Can you work these out from the model? Positions are in its coordinate system, mm. Face numbers are marked on the shaded views. Coordinates: 2 decimals unless noted, no trailing zeros. Loops run counter-clockwise (first coordinate to the right, second up) from the corner with the lowest first, then second, coordinate; pieces in that order, holes last.
```python
from build123d import *

# Parameters (mm, degrees)
SKETCH_1_R      = 13.5
SKETCH_1_R_2    = 10
EXTRUDE_1_DEPTH = 4


with BuildPart() as part:
    # 草图1 → 凸台-拉伸1 (new body)
    with BuildSketch(Plane(origin=(0, 0, 0), x_dir=(1, 0, 0), z_dir=(0, 1, 0))):
        with Locations(Location((0, 0, 0), (0, 0, 270))):
            Circle(SKETCH_1_R)
        with Locations(Location((0, 0, 0), (0, 0, 270))):
            Circle(SKETCH_1_R_2, mode=Mode.SUBTRACT)
    extrude(amount=EXTRUDE_1_DEPTH)

    # 草图3 → 切除-旋转1 (revolve, cut)
    with BuildSketch(Plane.XY, mode=Mode.PRIVATE) as cut_revolve_1_sk:
        Polygon((-12.25, 3.566987298), (-12, 4), (-12.5, 4), align=None)
        Polygon((-10.75, 3.566987298), (-10.5, 4), (-11, 4), align=None)
    cut_revolve_1 = revolve(cut_revolve_1_sk.sketch.rotate(Axis((0, 4, 0), (0, 1, 0)), 270), axis=Axis((0, 4, 0), (0, 1, 0)), mode=Mode.SUBTRACT)

    # 镜向1: 切除-旋转1 across plane
    add(cut_revolve_1.mirror(Plane.ZX.offset(2)), mode=Mode.SUBTRACT)


solid = part.part
```
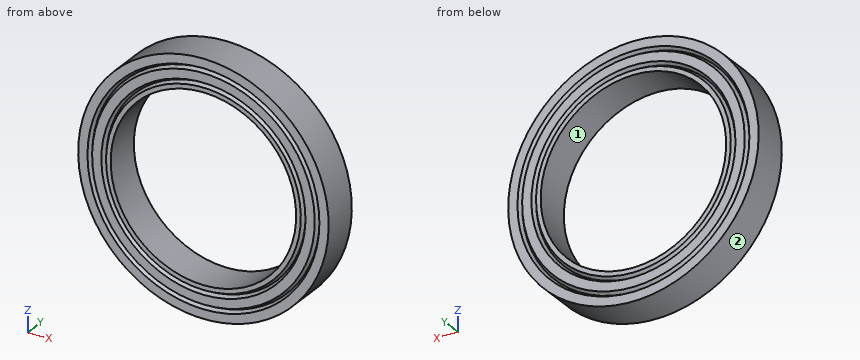
Item 1: I'm going to push a flat-ended pin straight in: P1, Ø1.5, axis at x = 9, y = 2, coming from the +Z side. Where does the tip first touch, or does it pass through?
Results are:
P1: stops at z = 10.69
Item 2: I need wall thicknesses on line 1 along Z through (x, y) = (5, 0.2); line 2 along X through (y, z) = (1, 0); line 3 along X through (y, z) = (3.3, 4.5). Which ranges of each line are inside material? Lowest first, please.
Results are:
line 1: z = -12.54 to -11.33, -11.04 to -9.67, -9.36 to -8.66, 8.66 to 9.36, 9.67 to 11.04, 11.33 to 12.54
line 2: x = -13.5 to -10, 10 to 13.5
line 3: x = -12.73 to -8.93, 8.93 to 12.73
Item 3: Suppose I cut it at C-C, the plane y = 2.7. Please give me the cut outline in (x, z).
Results are:
outline: circle Ø27 at (0, 0); hole circle Ø20 at (0, 0)
Item 4: We'd pull the mould along X, two halves only. Please class the marked faces 1 and 2: +X half, -X half, draft (parallel to the pull), parting line (faces both ways), or undercut.
Results are:
face 1: undercut
face 2: parting line
